Read the model definition and answer for the solid it produces. Units are mm, in the model's axes. A direction names the side the tool comes from. Give positions to 0.01 mm unless a question says otherwise; leave off trailing zeros. Order: outer loops, then holes, each group sorted by start corner. A loop starts at its lowest first (then second) coordinate and runs counter-clockwise, first axis right, second up.
Item 1: A cutting plane is placed at B-B (y = 2.75). Write down the section's boundary in (x, z), plus the area to 3 significant figures.
Item 2: A cutting plane is placed at C-C (z = 1.75). Write down the section's boundary in (x, y), plus the area to 3 significant figures.
Item 3: A cutting plane is placed at A-A (x = 0). Write down the section's boundary in (y, z), plus the area to 4 significant figures.
Item 4: Which of the six approach directions +Z, -Z, +X, -X, +Y, -Y give full straight-line access (tool end or side, diameter ignored) to faces 1 (the face through (3, 27, 1.8)), 2 (the face through (-2, 25, 2))?
Item 5: Given pin 1 Ø1 at (y, z) = (3.5, -2.5) entering from -X; pin 2 Ø1 at (y, z) = (4, -0.5) entering from -X; pin 3 Ø3 at (x, y) = (2, 8) entering from -Z, each flat-ended and moving along its own axis, determine where each tip first touches the part or whether it passes through.
Item 6: A cutting plane is placed at D-D (x = 3). Write down the section's boundary in (y, z), plus the area to 3 significant figures.
Item 7: Find the intervals of material crossed by line 1 along Y through (x, z) = (-3.25, 0.5); line 2 along X through (y, z) = (4, 1); line 3 along X through (y, z) = (14.25, 0), in increasing order.
from build123d import *

# Parameters (mm, degrees)
SKETCH1_R           = 2.25
BOSS_EXTRUDE1_DEPTH = 25
SKETCH2_R           = 2.25
BOSS_EXTRUDE2_DEPTH = 4


with BuildPart() as part:
    # Sketch1 → Boss-Extrude1 (new body)
    with BuildSketch(Plane(origin=(0, 0, 0), x_dir=(1, 0, 0), z_dir=(0, 1, 0))):
        with Locations(Location((0, 0, 0), (0, 0, 270))):
            Circle(SKETCH1_R)
    extrude(amount=BOSS_EXTRUDE1_DEPTH)

    # Sketch2 → Boss-Extrude2 (add)
    with BuildSketch(Plane(origin=(0, 25, 0), x_dir=(1, 0, 0), z_dir=(0, 1, 0))):
        with Locations(Location((0, 0, 0), (0, 0, 270))):
            Circle(SKETCH2_R)
        Polygon((-4.041451884, 0), (4.041451884, 0), (2.020725942, 3.5), (-2.020725942, 3.5), align=None)
        Polygon((-2.020725942, -3.5), (2.020725942, -3.5), (4.041451884, 0), (-4.041451884, 0), align=None)
        with BuildLine():
            ThreePointArc((-2.25, 0), (0, -2.25), (2.25, 0))
            Line((2.25, 0), (-2.25, 0))
        make_face()
        with BuildLine():
            Line((-2.25, 0), (2.25, 0))
            ThreePointArc((2.25, 0), (0, 2.25), (-2.25, 0))
        make_face()
    extrude(amount=BOSS_EXTRUDE2_DEPTH)

    # Sketch5 → Cut-Revolve1 (revolve, cut)
    with BuildSketch(Plane.XY):
        Polygon((3.641451884, 29), (4.041451884, 29), (4.041451884, 28.6), align=None)
    revolve(axis=Axis((0, 29, 0), (0, -1, 0)), mode=Mode.SUBTRACT)


solid = part.part
Response values:
1. outline: circle Ø4.5 at (0, 0)
1. area: 15.9 mm2
2. outline: (-3.03, 25) - (-1.41, 25) - (-1.41, 0) - (1.41, 0) - (1.41, 25) - (3.03, 25) - (3.03, 29) - (-3.03, 29) - close
2. area: 95.0 mm2
3. outline: (0, -2.25) - (25, -2.25) - (25, -3.5) - (29, -3.5) - (29, 3.5) - (25, 3.5) - (25, 2.25) - (0, 2.25) - close
3. area: 140.5 mm2
4. face 1: +Z, +X, +Y, -Y
4. face 2: -Y
5. pin 1: stops at x = -1.03
5. pin 2: stops at x = -2.25
5. pin 3: stops at z = -2.19
6. outline: (25, -1.8) - (29, -1.8) - (29, 1.8) - (25, 1.8) - close
6. area: 14.4 mm2
7. line 1: y = 25 to 29
7. line 2: x = -2.02 to 2.02
7. line 3: x = -2.25 to 2.25
